from build123d import *

# Parameters (mm, degrees)
F0_R     = 49.0283190444
F1_DEPTH = 76.2
F2_R     = 37.255304708
F3_DEPTH = 152.4
F4_R     = 23.611936081
F5_DEPTH = 273


# Not quite as in the source:
# - an extrude ends at something that could not be found from the text; its depth is read off the source's solid


with BuildPart() as f1:
    # F0 (on Front) → F1 (new body)
    with BuildSketch(Plane.XZ):
        Circle(F0_R)
    extrude(amount=F1_DEPTH)

    # F2 (on Front) → F3 (join)
    with BuildSketch(Plane.XZ):
        Circle(F2_R)
    extrude(amount=F3_DEPTH)

    # F4 (on Front) → F5 (cut, through all)
    with BuildSketch(Plane.XZ):
        Circle(F4_R)
    extrude(amount=-F5_DEPTH, mode=Mode.SUBTRACT)


solid = f1.part
For this review, take the finished solid that the model builds, in its own axes (mm). A direction names the side the tool comes from. Round coordinates to 2 decimals unless told otherwise and drop trailing zeros. Write each loop counter-clockwise with the first axis right and the second up, starting at its lowest first coordinate (ties: lowest second). Pieces come first, ordered by that corner, then holes. Notation, with made-up numbers: M -21,46.25 L 9,46.25 A5 cw 9,54.25 Z; hole C -9.75,61.5 d1. An arc over 180 degrees is marked long. Write item = value, one per line. Start each with the question number.
(1) For line 1 along Y through (x, z) = (22.5, -37.5); line 2 along X through (y, z) = (-141.5, -12); line 3 along X through (y, z) = (-96, -18), list the stretches that pass through material, from the lowest coordinate up.
(2) We need section B-B (z = 9). Give the boundary of the cut face in (x, y).
(3) We need section C-C (y = -51). Give the boundary of the cut face in (x, z).
(4) We need section D-D (y = -126). Give the boundary of the cut face in (x, z), then the cut area to 3 significant figures.
(5) For faces 1 (the face through (26.36, -37.57, 41.34)), 2 (the face through (20.028, -113.767, 31.414)), list the 3-axis set-ups (+Z, -Z, +X, -X, +Y, -Y) from which the entire face can be reached by the end or side of a thin tool; tool diameter is ignored.
(6) We need section A-A (x = 0). Give the boundary of the cut face in (y, z), then the cut area to 3 significant figures.
(7) Clearance check with flat-ended pins moving along their axes: pin 1 Ø6 at (y, z) = (-44, 4.5) entering from +X; pin 2 Ø2 at (y, z) = (-95.5, 6.5) entering from +X; pin 3 Ø6 at (y, z) = (-123.5, -12.5) entering from +X. State where each tip first meets the part, or that it passes through.
Results found:
q1.line_1 = -76.2 to 0
q1.line_2 = -35.27 to 35.27
q1.line_3 = -32.62 to 32.62
q2.outline = M -48.2,-76.2 L -36.15,-76.2 L -36.15,-152.4 L 36.15,-152.4 L 36.15,-76.2 L 48.2,-76.2 L 48.2,0 L -48.2,0 Z
q3.outline = C 0,0 d98.06
q4.outline = C 0,0 d74.51
q4.area = 4,360 mm²
q5.face_1 = +Y, -Y
q5.face_2 = -Y
q6.outline = M -152.4,-37.26 L -76.2,-37.26 L -76.2,-49.03 L 0,-49.03 L 0,49.03 L -76.2,49.03 L -76.2,37.26 L -152.4,37.26 Z
q6.area = 13,100 mm²
q7.pin_1 = 49.01
q7.pin_2 = 36.85
q7.pin_3 = 36.02
